```python
from build123d import *

# Parameters (mm, degrees)
CROQUIS1_R                   = 25.47
SALIENTE_EXTRUIR1_DEPTH      = 7.5
CROQUIS2_R                   = 27.97
SALIENTE_EXTRUIR2_DEPTH      = 0.5
SALIENTE_EXTRUIR3_START      = -14.5
CROQUIS2_2_R                 = 27.97
SALIENTE_EXTRUIR3_DEPTH      = 0.5
CROQUIS3_R                   = 19
SALIENTE_EXTRUIR4_DEPTH      = 21
CORTAR_EXTRUIR1_DEPTH        = 45.552124528
CORTAR_EXTRUIR1_DEPTH_BACK   = 45.552124528
CROQUIS4_R                   = 4
CORTAR_EXTRUIR2_START        = -10.5
CROQUIS5_R                   = 19
CORTAR_EXTRUIR2_DEPTH        = 10.5
TALADRO_DE_MARGEN_PARA_M31_D = 3.4


with BuildPart() as part:
    # Croquis1 → Saliente-Extruir1 (new, symmetric)
    with BuildSketch(Plane(origin=(0, 0, 0), x_dir=(-1, 0, 0), z_dir=(0, 1, 0))):
        with Locations(Location((0, 0, 0), (0, 0, 90))):
            Circle(CROQUIS1_R)
    extrude(amount=SALIENTE_EXTRUIR1_DEPTH, both=True)

    # Croquis2 → Saliente-Extruir2 (add)
    with BuildSketch(Plane(origin=(0, 7.5, 0), x_dir=(-1, 0, 0), z_dir=(0, 1, 0))):
        with Locations(Location((0, 0, 0), (0, 0, 90))):
            Circle(CROQUIS2_R)
    extrude(amount=-SALIENTE_EXTRUIR2_DEPTH)

    # Croquis2<2> → Saliente-Extruir3 (add)
    with BuildSketch(Plane(origin=(0, 7.5, 0), x_dir=(-1, 0, 0), z_dir=(0, 1, 0)).offset(SALIENTE_EXTRUIR3_START)):
        with Locations(Location((0, 0, 0), (0, 0, 90))):
            Circle(CROQUIS2_2_R)
    extrude(amount=-SALIENTE_EXTRUIR3_DEPTH)

    # Croquis3 → Saliente-Extruir4 (add)
    with BuildSketch(Plane(origin=(0, -7.5, 0), x_dir=(-1, 0, 0), z_dir=(0, 1, 0))):
        with Locations(Location((0, 0, 0), (0, 0, 270))):
            Circle(CROQUIS3_R)
    extrude(amount=SALIENTE_EXTRUIR4_DEPTH)

    # Croquis4 → Cortar-Extruir1 (cut, two sides: drawn at the far end of the back side and taken through both)
    with BuildSketch(Plane(origin=(0, -7, 0), x_dir=(-1, 0, 0), z_dir=(0, 1, 0)).offset(-CORTAR_EXTRUIR1_DEPTH_BACK)):
        with Locations(Location((0, 0, 0), (0, 0, 90))):
            Circle(CROQUIS4_R)
    extrude(amount=CORTAR_EXTRUIR1_DEPTH + CORTAR_EXTRUIR1_DEPTH_BACK, mode=Mode.SUBTRACT)

    # Croquis5 → Cortar-Extruir2 (cut)
    with BuildSketch(Plane(origin=(0, 13.5, 0), x_dir=(-1, 0, 0), z_dir=(0, 1, 0)).offset(CORTAR_EXTRUIR2_START)):
        with Locations(Location((0, 0, 0), (0, 0, 90))):
            Circle(CROQUIS5_R)
    cortar_extruir2 = extrude(amount=CORTAR_EXTRUIR2_DEPTH, mode=Mode.SUBTRACT)

    # Simetría1: Cortar-Extruir2 across plane
    add(cortar_extruir2.mirror(Plane.ZX), mode=Mode.SUBTRACT)

    # Taladro de margen para M31 (through all)
    with Locations(Plane(origin=(0, 7.5, 0), x_dir=(-1, 0, 0), z_dir=(0, 1, 0))):
        with Locations((0, 0), (9, 0), (-4.5, -7.794228634), (-4.5, 7.794228634)):
            Hole(TALADRO_DE_MARGEN_PARA_M31_D / 2)


solid = part.part
```
Check sheet for the modelled part. Datum: model origin and axes. Units: mm. A direction names the side the tool comes from. Coordinates: 2 decimals unless noted, no trailing zeros. Order: outer loops, then holes, each group sorted by start corner. A loop starts at its lowest first (then second) coordinate and runs counter-clockwise, first axis right, second up. Notation, with made-up numbers: (41.25, 15) -> (80.25, 15) arc R24 cw to (80.25, 35) -> close; hole circle Ø1 at (-35, 64). An arc over 180 degrees is marked (long way). Write each question's results on one line, items separated by ' | '. Start each with the question number.
1) Section check B-B (z = 0). Enter the section's corners in (x, y).
2) Depth check by flat-ended pin: pin 1 (6.5 mm diameter, centred on x = 0, z = 0, fed in from -Y); pin 2 (5 mm diameter, centred on y = -2, z = 10.5, fed in from +X); pin 3 (4.5 mm diameter, centred on x = -9, z = 0, fed in from +Y); pin 4 (8 mm diameter, centred on x = 5, y = 2.5, fed in from -Z). Enter the tip coordinate at first touch or a pass-through.
3) Section check C-C (z = -17.5). Enter the section's corners in (x, y), and give its area (3 significant figures).
4) Set-up check for faces 4 (the face through (4.5, 3, -0.3)), 5 (the face through (-11.56, -5.22, -15.08)), 6 (the face through (15, -7, -21)): record each of +Z, -Z, +X, -X, +Y, -Y from which the full face is reachable in a straight line by a thin tool's end or side.
5) Section check A-A (x = 0). Enter the section's corners in (y, z), and give its area (3 significant figures).
6) Draft check along Z on faces 1 (the face through (15, 7, -21)), 2 (the face through (6.07, -0.04, 7.14)), 3 (the face through (-27.305, 7.254, -6.063)). Enter one of: pulls with the +Z half, pulls with the -Z half, needs draft (parallel to the pull), parting line crosses it, or undercut.
7) Material ranges on line 1 along Y through (x, z) = (-8, -25); line 2 along Y through (x, z) = (9, 13.5); line 3 along X through (y, z) = (-3.9, 0), recorded low to high.
8) Section check D-D (x = 15). Enter the section's corners in (y, z), and give its area (3 significant figures).
Checked values:
1) outline: (-27.97, -7.5) -> (-19, -7.5) -> (-19, -3) -> (-10.7, -3) -> (-10.7, 3) -> (-19, 3) -> (-19, 7.5) -> (-27.97, 7.5) -> (-27.97, 7) -> (-25.47, 7) -> (-25.47, -7) -> (-27.97, -7) -> close; (-7.3, -3) -> (-4, -3) -> (-4, 3) -> (-7.3, 3) -> close; (4, -3) -> (19, -3) -> (19, -7.5) -> (27.97, -7.5) -> (27.97, -7) -> (25.47, -7) -> (25.47, 7) -> (27.97, 7) -> (27.97, 7.5) -> (19, 7.5) -> (19, 3) -> (4, 3) -> close
2) pin 1: through | pin 2: x = 24.18 | pin 3: y = 3 | pin 4: z = -25.45
3) outline: (-21.82, -7.5) -> (-7.4, -7.5) -> (-7.4, -3) -> (7.4, -3) -> (7.4, -7.5) -> (21.82, -7.5) -> (21.82, -7) -> (18.51, -7) -> (18.51, 7) -> (21.82, 7) -> (21.82, 7.5) -> (7.4, 7.5) -> (7.4, 3) -> (-7.4, 3) -> (-7.4, 7.5) -> (-21.82, 7.5) -> (-21.82, 7) -> (-18.51, 7) -> (-18.51, -7) -> (-21.82, -7) -> close | area: 429 mm²
4) face 4: +Y | face 5: -Y | face 6: none
5) outline: (-7.5, -27.97) -> (-7, -27.97) -> (-7, -25.47) -> (7, -25.47) -> (7, -27.97) -> (7.5, -27.97) -> (7.5, -19) -> (3, -19) -> (3, -4) -> (-3, -4) -> (-3, -19) -> (-7.5, -19) -> close; (-7.5, 19) -> (-3, 19) -> (-3, 4) -> (3, 4) -> (3, 19) -> (7.5, 19) -> (7.5, 27.97) -> (7, 27.97) -> (7, 25.47) -> (-7, 25.47) -> (-7, 27.97) -> (-7.5, 27.97) -> close | area: 379 mm²
6) face 1: needs draft | face 2: undercut | face 3: parting line crosses it
7) line 1: -7.5 to -7, 7 to 7.5 | line 2: -3 to 3 | line 3: -25.47 to -19, 19 to 25.47
8) outline: (-7.5, -23.61) -> (-7, -23.61) -> (-7, -20.58) -> (7, -20.58) -> (7, -23.61) -> (7.5, -23.61) -> (7.5, -11.66) -> (3, -11.66) -> (3, 11.66) -> (7.5, 11.66) -> (7.5, 23.61) -> (7, 23.61) -> (7, 20.58) -> (-7, 20.58) -> (-7, 23.61) -> (-7.5, 23.61) -> (-7.5, 11.66) -> (-3, 11.66) -> (-3, -11.66) -> (-7.5, -11.66) -> close | area: 414 mm²
